```python
from build123d import *

# Parameters (mm, degrees)
F0_W     = 25.4
F0_H     = 25.4
F0_R     = 1.5875
F1_DEPTH = 4.7625
F2_R     = 6.35


with BuildPart() as f1:
    # F0 (on Top) → F1 (new body)
    with BuildSketch(Plane.XY):
        with Locations((0, 12.7)):
            Rectangle(F0_W, F0_H)
        with Locations((0, 17.4625)):
            Circle(F0_R, mode=Mode.SUBTRACT)
    extrude(amount=F1_DEPTH)

    # F2
    f2_edges = [f1.edges().sort_by_distance(p)[0] for p in [
        (-12.7, 25.4, 2.38125),
        (12.7, 25.4, 2.38125),
    ]]
    fillet(f2_edges, radius=F2_R)


solid = f1.part
```
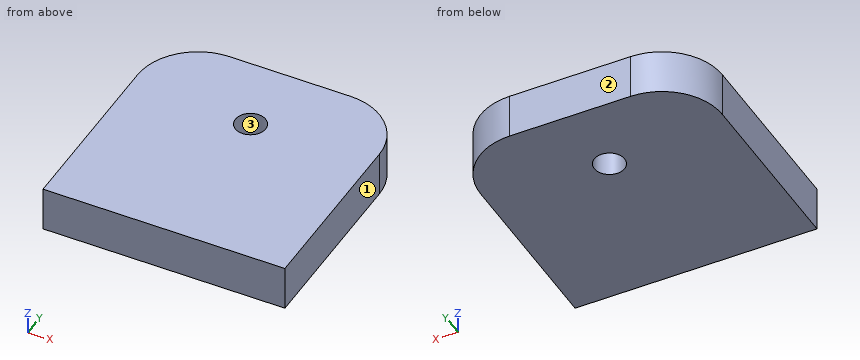
CAD build for the part. Positions are in the model's coordinates, mm. Face numbers are marked on the shaded views. Give positions to 0.01 mm unless a question says otherwise; leave off trailing zeros. Write each loop counter-clockwise with the first axis right and the second up, starting at its lowest first coordinate (ties: lowest second). Pieces come first, ordered by that corner, then holes. Notation, with made-up numbers: M 83,-11 L 110,-11 A21 cw 110,18 Z; hole C 73.25,40 d10. An arc over 180 degrees is marked long. Return JSON: item names as keys, results as strings. Group by question number.
(1) Band-saw the part on C-C (x = 10.5). Give the cut face in (y, z).
(2) Drill centre lines: L1, parallel to Y at x = 0, z = 3 (3 decimals); L2, parallel to X at y = 19.25, z = 3.9; L3, parallel to X at y = 23.25, z = 1.1. Where is each one in solid material? Low to high. Write a range as [from, to].
(3) Mould opens along X. For the marked faces 1, 2 and 3 say: pulls with the +X half, pulls with the -X half, needs draft (parallel to the pull), parting line crosses it, or undercut.
(4) Flat gauge pins, fed straight in: pin 1 Ø1 at (y, z) = (20.5, 0.5) entering from -X; pin 2 Ø2 at (y, z) = (20, 4) entering from -X. Where does each tip first touch, or does it go through?
Entries:
{
 "1": {"outline": "M 0,0 L 23.86,0 L 23.86,4.76 L 0,4.76 Z"},
 "2": {"L1": "y = [0, 15.875], [19.05, 25.4]", "L2": "x = [-12.7, 12.7]", "L3": "x = [-11.11, 11.11]"},
 "3": {"face 1": "pulls with the +X half", "face 2": "needs draft", "face 3": "undercut"},
 "4": {"pin 1": "stops at x = -12.63", "pin 2": "stops at x = -12.7"}
}
